Check sheet for the modelled part. Datum: model origin and axes. Units: mm. Face numbers are marked on the shaded views. A direction names the side the tool comes from. Round coordinates to 2 decimals unless told otherwise and drop trailing zeros. Write each loop counter-clockwise with the first axis right and the second up, starting at its lowest first coordinate (ties: lowest second). Pieces come first, ordered by that corner, then holes.
Item 1: Depth check by flat-ended pin: pin 1 (5 mm diameter, centred on y = 13.5, z = 8.5, fed in from +X); pin 2 (0.8 mm diameter, centred on y = 34, z = 3.5, fed in from -X) (3 decimals); pin 3 (0.6 mm diameter, centred on x = 26.5, z = 6.5, fed in from +Y). Enter the tip coordinate at first touch or a pass-through.
Item 2: Set-up check for the marked faces 1, 2 and 3: record each of +Z, -Z, +X, -X, +Y, -Y from which the full face is reachable in a straight line by a thin tool's end or side.
Item 3: Release check for a two-part mould opening along Y. For the marked faces 4, 5 and 6 record: pulls with the +Y half, pulls with the -Y half, needs draft (parallel to the pull), parting line crosses it, or undercut.
Item 4: Section check A-A, the plane x = 0. Record the cut outline in (y, z), plus the area to 3 significant figures.
Item 5: Material ranges on line 1 along X through (y, z) = (22, 5.5); line 2 along X through (y, z) = (23, 5); line 3 along Y through (x, z) = (0, 7.25), recorded low to high.
from build123d import *

# Parameters (mm, degrees)
F1_DEPTH    = 12
F3_D        = 5.5
F3_DEPTH    = 7
F3_TIP      = 1.6523667023
F4_T1_DEPTH = 12
F4_T3_DEPTH = 27
F4_T5_DEPTH = 17.1641728771
F4_T7_DEPTH = 19.3168092608
F4_T9_DEPTH = 21.2169428411


# Not quite as in the source:
# - a fillet or chamfer that OpenCascade refuses, or shapes differently, is made with other operations: its cross-section is extruded or revolved along the edge and cut away or added
# - a feature names something its author has since deleted; it is built from what else it names


with BuildPart() as f1:
    # F0 (on Top) → F1 (new body)
    with BuildSketch(Plane.XY):
        with BuildLine():
            Line((5.4365318258, 35.1470746964), (5.4365318258, 33.4868409083))
            Line((5.4365318258, 33.4868409083), (3.5, 33.4868409083))
            ThreePointArc((3.5, 33.4868409083), (0, 29.9868409083), (-3.5, 33.4868409083))
            Line((-3.5, 33.4868409083), (-5.4365318258, 33.4868409083))
            Line((-5.4365318258, 33.4868409083), (-5.4365318258, 35.1470746964))
            Line((-5.4365318258, 35.1470746964), (-8.2365318258, 35.1470746964))
            Line((-8.2365318258, 35.1470746964), (-17.1626134825, 23.7201299491))
            Line((-17.1626134825, 23.7201299491), (-14.2073691514, 21.4116605551))
            Line((-14.2073691514, 21.4116605551), (-12.8128593238, 23.1968768865))
            Line((-12.8128593238, 23.1968768865), (-10.5274703744, 21.4116605551))
            Line((-10.5274703744, 21.4116605551), (-15.298307122, 15.304155604))
            Line((-15.298307122, 15.304155604), (-17.5836960714, 17.0893719354))
            Line((-17.5836960714, 17.0893719354), (-15.9925854827, 19.1262716057))
            Line((-15.9925854827, 19.1262716057), (-18.9478298139, 21.4347409997))
            Line((-18.9478298139, 21.4347409997), (-25.5365714751, 13))
            Line((-25.5365714751, 13), (-25.5365714751, 0))
            Line((-25.5365714751, 0), (-25.5365714751, -4))
            Line((-25.5365714751, -4), (-20.5365714751, -4))
            Line((-20.5365714751, -4), (-15.3852878138, -4))
            Line((-15.3852878138, -4), (-15.3852878138, -2.5156375486))
            Line((-15.3852878138, -2.5156375486), (-20.5365714751, 0))
            Line((-20.5365714751, 0), (-20.5365714751, 4.3))
            Line((-20.5365714751, 4.3), (-17.6668407531, 4.3))
            Line((-17.6668407531, 4.3), (-3.9629505379, 10.990731871))
            ThreePointArc((-3.9629505379, 10.990731871), (0, 18.1703798791), (3.9629505379, 10.990731871))
            Line((3.9629505379, 10.990731871), (17.6668407531, 4.3))
            Line((17.6668407531, 4.3), (20.5365714751, 4.3))
            Line((20.5365714751, 4.3), (20.5365714751, -4))
            Line((20.5365714751, -4), (30.5365714751, -4))
            Line((30.5365714751, -4), (30.5365714751, 0))
            Line((30.5365714751, 0), (25.5365714751, 0))
            Line((25.5365714751, 0), (25.5365714751, 13))
            Line((25.5365714751, 13), (18.9478298139, 21.4347409997))
            Line((18.9478298139, 21.4347409997), (15.9925854827, 19.1262716057))
            Line((15.9925854827, 19.1262716057), (17.5836960714, 17.0893719354))
            Line((17.5836960714, 17.0893719354), (15.298307122, 15.304155604))
            Line((15.298307122, 15.304155604), (10.5274703744, 21.4116605551))
            Line((10.5274703744, 21.4116605551), (12.8128593238, 23.1968768865))
            Line((12.8128593238, 23.1968768865), (14.2073691514, 21.4116605551))
            Line((14.2073691514, 21.4116605551), (17.1626134825, 23.7201299491))
            Line((17.1626134825, 23.7201299491), (8.2365318258, 35.1470746964))
            Line((8.2365318258, 35.1470746964), (5.4365318258, 35.1470746964))
        make_face()
    extrude(amount=F1_DEPTH)

    # F3
    with Locations(Plane(origin=(-22.1660473582, 17.3148600175, 0), x_dir=(-0.6155918384, -0.788065155, 0), z_dir=(-0.788065155, 0.6155918384, 0))):
        with Locations((-15.1406489313, 6.5862988122)):
            Hole(F3_D / 2, depth=F3_DEPTH)
            with Locations((0, 0, -(F3_DEPTH + F3_TIP / 2))):  # 118° drill point
                Cone(0, F3_D / 2, F3_TIP, mode=Mode.SUBTRACT)

    # F4: fillet of radius 3 on 10 edges, made by hand

    # F4_s2 → F4_t1 (join)
    with BuildSketch(Plane.XY):
        with BuildLine():
            ThreePointArc((17.6668407531, 4.3), (19.7034595472, 3.3775817354), (20.5365714751, 1.302829682))
            Line((20.5365714751, 1.302829682), (20.5365714751, 4.3))
            Line((20.5365714751, 4.3), (17.6668407531, 4.3))
        make_face()
    extrude(amount=F4_T1_DEPTH)

    # F4_s4 → F4_t3 (cut)
    with BuildSketch(Plane.XY.offset(-7.5)):
        with BuildLine():
            ThreePointArc((20.5365714751, -1), (21.4152511315, -3.1213203436), (23.5365714751, -4))
            Line((23.5365714751, -4), (20.5365714751, -4))
            Line((20.5365714751, -4), (20.5365714751, -1))
        make_face()
        with BuildLine():
            ThreePointArc((-25.5365714751, -1), (-24.6578918186, -3.1213203436), (-22.5365714751, -4))
            Line((-22.5365714751, -4), (-25.5365714751, -4))
            Line((-25.5365714751, -4), (-25.5365714751, -1))
        make_face()
        with BuildLine():
            ThreePointArc((30.5365714751, -3), (29.6578918186, -0.8786796564), (27.5365714751, 0))
            Line((27.5365714751, 0), (30.5365714751, 0))
            Line((30.5365714751, 0), (30.5365714751, -3))
        make_face()
        with BuildLine():
            ThreePointArc((27.5365714751, -4), (29.6578918186, -3.1213203436), (30.5365714751, -1))
            Line((30.5365714751, -1), (30.5365714751, -4))
            Line((30.5365714751, -4), (27.5365714751, -4))
        make_face()
    extrude(amount=F4_T3_DEPTH, mode=Mode.SUBTRACT)

    # F4_s6 → F4_t5 (cut)
    with BuildSketch(Plane.XY.offset(-2.5820864386)):
        with BuildLine():
            ThreePointArc((25.5365714751, 11.9671654246), (25.3731703536, 12.9437445573), (24.90076694, 13.8139409398))
            Line((24.90076694, 13.8139409398), (25.5365714751, 13))
            Line((25.5365714751, 13), (25.5365714751, 11.9671654246))
        make_face()
        with BuildLine():
            ThreePointArc((-24.90076694, 13.8139409398), (-25.3731703536, 12.9437445573), (-25.5365714751, 11.9671654246))
            Line((-25.5365714751, 11.9671654246), (-25.5365714751, 13))
            Line((-25.5365714751, 13), (-24.90076694, 13.8139409398))
        make_face()
    extrude(amount=F4_T5_DEPTH, mode=Mode.SUBTRACT)

    # F4_s8 → F4_t7 (cut)
    with BuildSketch(Plane.XY.offset(-3.6584046304)):
        with BuildLine():
            ThreePointArc((9.1373654386, 33.9938502116), (8.088402549, 34.843398726), (6.7731699737, 35.1470746964))
            Line((6.7731699737, 35.1470746964), (8.2365318258, 35.1470746964))
            Line((8.2365318258, 35.1470746964), (9.1373654386, 33.9938502116))
        make_face()
        with BuildLine():
            ThreePointArc((-6.7731699737, 35.1470746964), (-8.088402549, 34.843398726), (-9.1373654386, 33.9938502116))
            Line((-9.1373654386, 33.9938502116), (-8.2365318258, 35.1470746964))
            Line((-8.2365318258, 35.1470746964), (-6.7731699737, 35.1470746964))
        make_face()
    extrude(amount=F4_T7_DEPTH, mode=Mode.SUBTRACT)

    # F4_s10 → F4_t9 (cut)
    with BuildSketch(Plane.XY.offset(-4.6084714206)):
        with BuildLine():
            ThreePointArc((-15.3852878138, -4), (-15.9262171402, -2.6458583956), (-17.0417102945, -1.7067210022))
            Line((-17.0417102945, -1.7067210022), (-15.3852878138, -2.5156375486))
            Line((-15.3852878138, -2.5156375486), (-15.3852878138, -4))
        make_face()
    extrude(amount=F4_T9_DEPTH, mode=Mode.SUBTRACT)


solid = f1.part
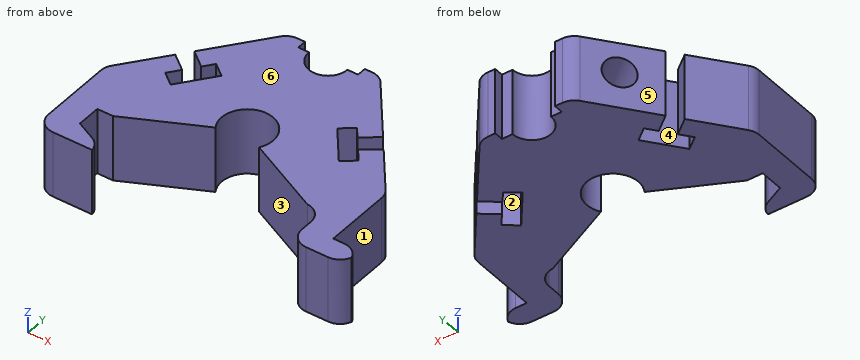
Values found:
1. pin 1: stops at x = 25.54
1. pin 2: stops at x = -9.445
1. pin 3: stops at y = 0
2. face 1: +Z, -Z, +X, +Y
2. face 2: +Z, -Z
2. face 3: +Z, -Z, -Y
3. face 4: undercut
3. face 5: pulls with the +Y half
3. face 6: needs draft
4. outline: (18.17, 0) - (29.99, 0) - (29.99, 12) - (18.17, 12) - close
4. area: 142 mm2
5. line 1: x = -14.96 to -13.75, -11.28 to 11.28, 13.75 to 14.96
5. line 2: x = -16.24 to -12.97, -12.56 to 12.56, 12.97 to 16.24
5. line 3: y = 18.17 to 29.99
